Job drawing, mm, ordinate dimensions from the low corner. One solid piece. Coordinates: 2 decimals unless noted, no trailing zeros. Loops run counter-clockwise (first coordinate to the right, second up) from the corner with the lowest first, then second, coordinate; pieces in that order, holes last. Notation, with made-up numbers: (54.25, 77.25) -> (105.25, 77.25) arc R21 cw to (105.25, 87.25) -> close; hole circle Ø11 at (0, 78.5). An arc over 180 degrees is marked (long way). Use one line per item in the form item = value. Start each with the question number.
(1) Band-saw the part on D-D on z = 8. Give the cut face in (x, y), then the cut area to 3 significant figures.
(2) Drill centre lines: L1, parallel to Y at x = 8.5, z = 4.75; L2, parallel to X at y = 9, z = 3.75; L3, parallel to X at y = 3.75, z = 1.25. Where is each one in solid material? Low to high. Write a range as [from, to].
(3) Band-saw the part on B-B on y = 5. Give the cut face in (x, z).
(4) Mould opens along X. For the marked faces 1, 2, 3 and 4 say: +X half, -X half, draft (parallel to the pull), parting line (faces both ways), or undercut.
(5) Band-saw the part on A-A on z = 5. Give the cut face in (x, y), then the cut area to 3 significant figures.
(6) Band-saw the part on C-C on x = 5. Give the cut face in (y, z), then the cut area to 3 significant figures.
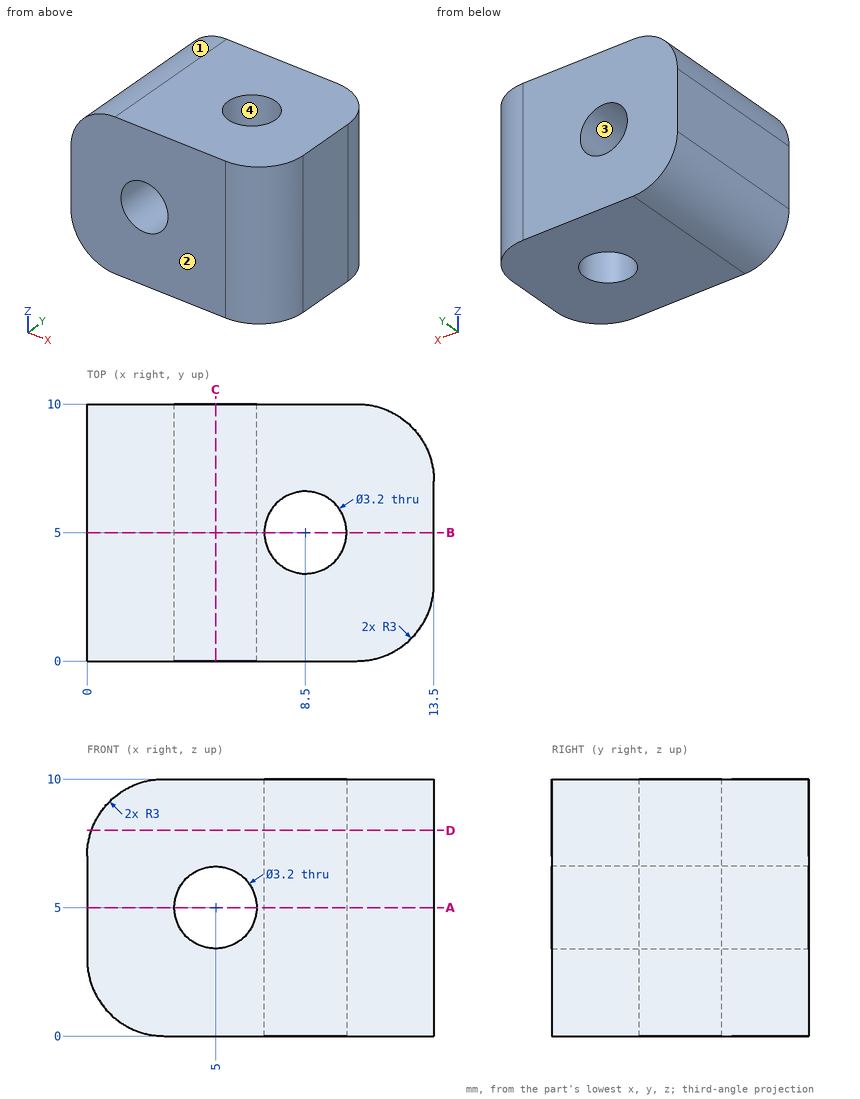
A:
q1.outline = (0.17, 0) -> (10.5, 0) arc R3 ccw to (13.5, 3) -> (13.5, 7) arc R3 ccw to (10.5, 10) -> (0.17, 10) -> close; hole circle Ø3.2 at (8.5, 5)
q1.area = 121 mm²
q2.L1 = [0, 3.4], [6.6, 10]
q2.L2 = [0, 4], [6, 12.74]
q2.L3 = [0.56, 7.5], [9.5, 13.5]
q3.outline = (0, 3) arc R3 ccw to (3, 0) -> (6.9, 0) -> (6.9, 10) -> (3, 10) arc R3 ccw to (0, 7) -> close; (10.1, 0) -> (13.5, 0) -> (13.5, 10) -> (10.1, 10) -> close; hole circle Ø3.2 at (5, 5)
q4.face_1 = -X half
q4.face_2 = draft
q4.face_3 = undercut
q4.face_4 = undercut
q5.outline = (0, 0) -> (3.4, 0) -> (3.4, 10) -> (0, 10) -> close; (6.6, 0) -> (10.5, 0) arc R3 ccw to (13.5, 3) -> (13.5, 7) arc R3 ccw to (10.5, 10) -> (6.6, 10) -> close; hole circle Ø3.2 at (8.5, 5)
q5.area = 91.1 mm²
q6.outline = (0, 0) -> (10, 0) -> (10, 3.4) -> (0, 3.4) -> close; (0, 6.6) -> (10, 6.6) -> (10, 10) -> (0, 10) -> close
q6.area = 68.0 mm²
